Autodesk Inventor part; units mm, degrees
ref_plane "YZ Plane" through (0, 0, 0) normal (1, 0, 0) x (0, 1, 0)
ref_plane "XZ Plane" through (0, 0, 0) normal (0, 1, 0) x (-1, 0, 0)
ref_plane "XY Plane" through (0, 0, 0) normal (0, 0, 1) x (1, 0, 0)
sketch "スケッチ1" plane through (0, 0, 0) normal (0, 0, 1) x (1, 0, 0)
  line L0 (0, 0) -> (8, 0)
  line L1 (8, 0) -> (8, 30)
  line L2 (8, 30) -> (0, 30)
  line L3 (0, 30) -> (0, 0)
  dimension "d0" = 8
  dimension "d1" = 30
extrude "押し出し1" add sketch "スケッチ1" along normal blind 3
sketch "スケッチ2" plane through (0, 0, 3) normal (0, 0, 1) x (1, 0, 0)
  line L0 (8, 0) -> (8, 30)
  line L1 (8, 30) -> (0, 30)
  line L2 (0, 0) -> (8, 0)
  point P0 (4, 25)
  point P1 (4, 5)
  dimension "d4" = 4
  dimension "d5" = 5
  dimension "d6" = 5
  dimension "d7" = 4
hole "穴1" at (4, 25, 3) at (4, 5, 3) direction (0, 0, -1) diameter 3.5 end through all
properties part number "3SR14_ポテンショメータ固定台"
Geometry: final body of the model. Coordinates: model frame, mm. Round coordinates to 2 decimals unless told otherwise and drop trailing zeros. Write each loop counter-clockwise with the first axis right and the second up, starting at its lowest first coordinate (ties: lowest second). Pieces come first, ordered by that corner, then holes. Notation, with made-up numbers: (32, 85) -> (51, 85) arc R4 cw to (51, 90) -> close; hole circle Ø7 at (-35.5, 52.25). An arc over 180 degrees is marked (long way). Use CSV: the item, a comma, the result in double quotes. Start each with the question number.
Q1. Section D-D (x = 2.75). Return loops of the section in (y, z).
Q2. Line query: L1, parallel to Y at x = 4, z = 0.9; L2, parallel to Y at x = 2.5, z = 1.8; L3, parallel to X at y = 5, z = 1.45. Output: solid intervals per line, ascending.
Q3. Section C-C (z = 1.4). Return loops of the section in (x, y), plus the area to 3 significant figures.
Q4. Pull-direction query (X, two-part tool) for faces 1 (the face through (4, 0, 1)), 2 (the face through (8, 15, 1)), 3 (the face through (3.92, 26.75, 1.48)); classes: pulls with the +X half, pulls with the -X half, needs draft (parallel to the pull), parting line crosses it, or undercut.
Q5. Section A-A (y = 5). Return loops of the section in (x, z).
Q6. Section B-B (x = 4). Return loops of the section in (y, z).
Result sheet:
1,outline,"(0, 0) -> (3.78, 0) -> (3.78, 3) -> (0, 3) -> close; (6.22, 0) -> (23.78, 0) -> (23.78, 3) -> (6.22, 3) -> close; (26.22, 0) -> (30, 0) -> (30, 3) -> (26.22, 3) -> close"
2,L1,"0 to 3.25, 6.75 to 23.25, 26.75 to 30"
2,L2,"0 to 4.1, 5.9 to 24.1, 25.9 to 30"
2,L3,"0 to 2.25, 5.75 to 8"
3,outline,"(0, 0) -> (8, 0) -> (8, 30) -> (0, 30) -> close; hole circle Ø3.5 at (4, 5); hole circle Ø3.5 at (4, 25)"
3,area,"221 mm²"
4,face 1,"needs draft"
4,face 2,"pulls with the +X half"
4,face 3,"undercut"
5,outline,"(0, 0) -> (2.25, 0) -> (2.25, 3) -> (0, 3) -> close; (5.75, 0) -> (8, 0) -> (8, 3) -> (5.75, 3) -> close"
6,outline,"(0, 0) -> (3.25, 0) -> (3.25, 3) -> (0, 3) -> close; (6.75, 0) -> (23.25, 0) -> (23.25, 3) -> (6.75, 3) -> close; (26.75, 0) -> (30, 0) -> (30, 3) -> (26.75, 3) -> close"
